Build history of the part. All positions in model axes, mm. A direction names the side the tool comes from. Give positions to 0.01 mm unless a question says otherwise; leave off trailing zeros. Order: outer loops, then holes, each group sorted by start corner. A loop starts at its lowest first (then second) coordinate and runs counter-clockwise, first axis right, second up. Notation, with made-up numbers: (-3, -24) - (9, -24) arc R19 ccw to (9, 2) - close; hole circle Ø7 at (74.5, -24). An arc over 180 degrees is marked (long way). Use a Markdown table: item, result. Add a question column.
(1) Flat gauge pins, fed straight in: pin 1 (10 mm diameter, centred on y = 13, z = 67.5, fed in from -X); pin 2 (1.9 mm diameter, centred on x = -62.5, y = 3.5, fed in from +Z); pin 3 (4 mm diameter, centred on x = 61, y = 12.5, fed in from +Z). Where does each tip first touch, or does it go through?
(2) Slice it at B-B (z = 70.5). Write the cut outline in (x, y), then the cut area to 3 significant figures.
(3) Slice it at D-D (x = -19.5). Write the cut outline in (y, z), then the cut area to 3 significant figures.
(4) Mould opens along Z. For faces 5 (the face through (1, 5, -56.701)), 6 (the face through (67, 3, 44.704)), 7 (the face through (-66, 15, 25.4)), 8 (the face through (-69, 12.7, 0)) say: +Z half, -Z half, draft (parallel to the pull), parting line (faces both ways), or undercut.
(5) Which spindle directions (+Z, -Z, +X, -X, +Y, -Y) get a long thin tool onto all of the face, cutting with end or side? Do faces 1 (the face through (-25.4, 15, -66)), 2 (the face through (52.891, 13, 0)), 3 (the face through (56.701, 5, 1)), 4 (the face through (0, 13, 52.891)). Say none if no direction does.
(6) Slice it at A-A (y = 9.25). Write the cut outline in (x, z), then the cut area to 3 significant figures.
(7) Wall check: line 1 (X direction, y = 12.5, z = 8); line 2 (Y direction, x = -7.5, z = 68.5); line 3 (Z direction, x = -8.5, y = 1.75). Give the ranges that are in metal, low to high.
(8) Slice it at C-C (x = -63). Write the cut outline in (y, z), then the cut area to 3 significant figures.
from build123d import *

# Parameters (mm, degrees)
SKETCH1_R         = 88.773
BASE_DEPTH        = 6.35
STOPPER_DEPTH     = 12.7
STOPPER_START     = -6.35
STOPPER_GAP_DEPTH = 13.7
CIRPATTERN1_COUNT = 4


with BuildPart() as part:
    # Sketch1 → Base (new body)
    with BuildSketch(Plane(origin=(0, 0, 0), x_dir=(1, 0, 0), z_dir=(0, 1, 0))):
        Circle(SKETCH1_R)
    extrude(amount=BASE_DEPTH)

    # Sketch2 → Stopper (add)
    with BuildSketch(Plane(origin=(0, 6.35, 0), x_dir=(1, 0, 0), z_dir=(0, 1, 0))):
        with BuildLine():
            Line((-25.4, -78.545162168), (-25.4, -52.891162168))
            Line((-25.4, -52.891162168), (0, -52.891162168))
            Line((0, -52.891162168), (25.4, -52.891162168))
            Line((25.4, -52.891162168), (25.4, -78.545162168))
            ThreePointArc((25.4, -78.545162168), (12.856892374, -81.542644172), (0, -82.55))
            ThreePointArc((0, -82.55), (-12.856892374, -81.542644172), (-25.4, -78.545162168))
        make_face()
    stopper = extrude(amount=STOPPER_DEPTH)

    # Sketch5 → Stopper Gap (cut, through all)
    with BuildSketch(Plane(origin=(0, 19.05, 0), x_dir=(1, 0, 0), z_dir=(0, 1, 0)).offset(STOPPER_START)):
        with BuildLine():
            Line((-44.704, -76.695488218), (-44.704, -56.701162168))
            Line((-44.704, -56.701162168), (0, -56.701162168))
            Line((0, -56.701162168), (44.704, -56.701162168))
            Line((44.704, -56.701162168), (44.704, -76.695488218))
            ThreePointArc((44.704, -76.695488218), (23.153368582, -85.700449545), (0, -88.773))
            ThreePointArc((0, -88.773), (-23.153368582, -85.700449545), (-44.704, -76.695488218))
        make_face()
    stopper_gap = extrude(amount=-STOPPER_GAP_DEPTH, mode=Mode.SUBTRACT)

    # CirPattern1: Stopper, Stopper Gap ×4 about axis
    cirpattern1_axis = Axis((0, 0, 0), (0, 1, 0))
    for i in range(1, CIRPATTERN1_COUNT):
        add(stopper.rotate(cirpattern1_axis, i * 360 / CIRPATTERN1_COUNT))
        add(stopper_gap.rotate(cirpattern1_axis, i * 360 / CIRPATTERN1_COUNT), mode=Mode.SUBTRACT)


solid = part.part
Solution:
| question | item | result |
|---|---|---|
| 1 | pin 1 | x = -25.4 |
| 1 | pin 2 | z = 63.97 |
| 1 | pin 3 | z = 25.4 |
| 2 | outline | (-53.95, 0) - (-44.7, 0) - (-44.7, 6.35) - (-53.95, 6.35) - close; (-25.4, 12.7) - (25.4, 12.7) - (25.4, 19.05) - (-25.4, 19.05) - close; (44.7, 0) - (53.95, 0) - (53.95, 6.35) - (44.7, 6.35) - close |
| 2 | area | 440 mm2 |
| 3 | outline | (0, -56.7) - (12.7, -56.7) - (12.7, -80.21) - (19.05, -80.21) - (19.05, -52.89) - (6.35, -52.89) - (6.35, 52.89) - (19.05, 52.89) - (19.05, 80.21) - (12.7, 80.21) - (12.7, 56.7) - (0, 56.7) - close |
| 3 | area | 1,120 mm2 |
| 4 | face 5 | -Z half |
| 4 | face 6 | undercut |
| 4 | face 7 | +Z half |
| 4 | face 8 | draft |
| 5 | face 1 | +Z, -Z, -X, +Y |
| 5 | face 2 | +Z, -Z, +Y |
| 5 | face 3 | +X, -Y |
| 5 | face 4 | +X, -X, +Y |
| 6 | outline | (-56.7, -25.4) - (-52.89, -25.4) - (-52.89, 25.4) - (-56.7, 25.4) - close; (-25.4, -56.7) - (25.4, -56.7) - (25.4, -52.89) - (-25.4, -52.89) - close; (-25.4, 52.89) - (25.4, 52.89) - (25.4, 56.7) - (-25.4, 56.7) - close; (52.89, -25.4) - (56.7, -25.4) - (56.7, 25.4) - (52.89, 25.4) - close |
| 6 | area | 774 mm2 |
| 7 | line 1 | -56.7 to -52.89, 52.89 to 56.7 |
| 7 | line 2 | 12.7 to 19.05 |
| 7 | line 3 | -56.7 to 56.7 |
| 8 | outline | (0, -62.54) - (6.35, -62.54) - (6.35, -44.7) - (0, -44.7) - close; (0, 44.7) - (6.35, 44.7) - (6.35, 62.54) - (0, 62.54) - close; (12.7, -25.4) - (19.05, -25.4) - (19.05, 25.4) - (12.7, 25.4) - close |
| 8 | area | 549 mm2 |
